Part model, mm, in its own coordinate system. Face numbers are marked on the shaded views. A direction names the side the tool comes from. Coordinates: 2 decimals unless noted, no trailing zeros. Order: outer loops, then holes, each group sorted by start corner. A loop starts at its lowest first (then second) coordinate and runs counter-clockwise, first axis right, second up.
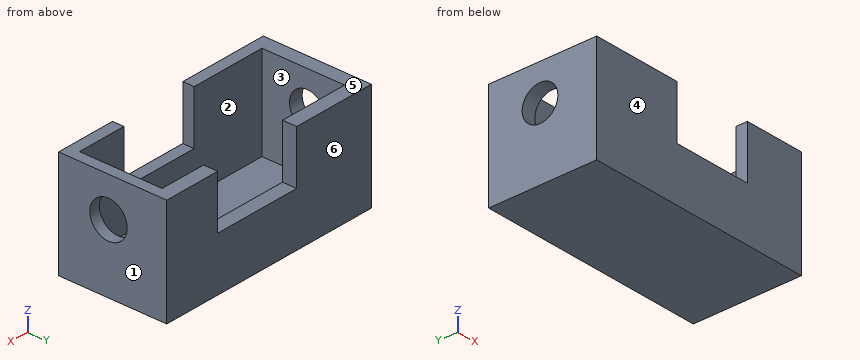
```python
from build123d import *

# Parameters (mm, degrees)
F0_W     = 218.6504378915
F0_H     = 102.5099009275
F1_DEPTH = 101.6
F2_W     = 194.8913782835
F2_H     = 78.3294849098
F3_DEPTH = 88.9
F4_W     = 84.4324864447
F4_H     = 13.4305804968
F4_W_2   = 74.9933160841
F4_H_2   = 10.749835521
F5_DEPTH = 50.8
F6_R     = 16.9313597919
F7_DEPTH = 25.4
F8_R     = 17.7291047607
F9_DEPTH = 25.4


with BuildPart() as f1:
    # F0 (on Top) → F1 (new body)
    with BuildSketch(Plane.XY):
        with Locations((-0.1867227256, -2.5207363069)):
            Rectangle(F0_W, F0_H)
    extrude(amount=F1_DEPTH)

    # F2 (on face) → F3 (cut)
    with BuildSketch(Plane.XY.offset(101.6)):
        with Locations((1.4596879482, -3.8611087948)):
            Rectangle(F2_W, F2_H)
    extrude(amount=-F3_DEPTH, mode=Mode.SUBTRACT)

    # F4 (on face) → F5 (cut)
    with BuildSketch(Plane.XY.offset(101.6)):
        with Locations((12.4733056873, 42.0189239085)):
            Rectangle(F4_W, F4_H)
        with Locations((13.9715243131, -48.4007690102)):
            Rectangle(F4_W_2, F4_H_2)
    extrude(amount=-F5_DEPTH, mode=Mode.SUBTRACT)

    # F6 (on face) → F7 (cut)
    with BuildSketch(Plane(origin=(-109.5119416714, 0, 0), x_dir=(0, -1, 0), z_dir=(-1, 0, 0))):
        with Locations((0, 67.3742890358)):
            Circle(F6_R)
    extrude(amount=-F7_DEPTH, mode=Mode.SUBTRACT)

    # F8 (on face) → F9 (cut)
    with BuildSketch(Plane.YZ.offset(109.1384962201)):
        with Locations((-6.4566782676, 64.2816573381)):
            Circle(F8_R)
    extrude(amount=-F9_DEPTH, mode=Mode.SUBTRACT)


solid = f1.part
```
(1) Pull direction Y, two halves, no side cores. Call the marked faces 3, 4, 5 and 6: +Y half, -Y half, draft (parallel to the pull), parting line (faces both ways), or undercut.
(2) Tool access for the marked faces 1 and 2: list every direction of +Z, -Z, +X, -X, +Y, -Y with a clear straight run to the whole face (end or side of a thin tool).
(3) Slice it at B-B, the plane y = -37.5. Give the cut face in (x, z), then the cut area to 3 significant figures.
(4) Slice it at D-D, the plane z = 30. Give the cut face in (x, y).
(5) Drop flat-ended pins along their axis: pin 1 (1.5 mm diameter, centred on y = 1, z = 77.5, fed in from -X); pin 2 (6.5 mm diameter, centred on x = -4, y = 45, fed in from +Z). Give the stop position or say it passes through.
(6) Slice it at C-C, the plane x = 40. Give the cut face in (y, z).
(7) Probe line 1 (Z direction, x = -104, y = 0); line 2 (Y direction, x = -69.5, z = 48); line 3 (X direction, y = 5, z = 20). List the from-to ranges inside material, lowest first.
(8) Slice it at A-A, the plane z = 73.5. Give the cut face in (x, y).
Here are the results:
1. face 3: undercut
1. face 4: -Y half
1. face 5: draft
1. face 6: +Y half
2. face 1: +Z, -Z, +X, +Y, -Y
2. face 2: +Z
3. outline: (-109.51, 0) - (109.14, 0) - (109.14, 101.6) - (98.91, 101.6) - (98.91, 12.7) - (-95.99, 12.7) - (-95.99, 101.6) - (-109.51, 101.6) - close
3. area: 4,890 mm2
4. outline: (-109.51, -53.78) - (109.14, -53.78) - (109.14, 48.73) - (-109.51, 48.73) - close; hole (-95.99, -43.03) - (98.91, -43.03) - (98.91, 35.3) - (-95.99, 35.3) - close
5. pin 1: passes through
5. pin 2: stops at z = 50.8
6. outline: (-53.78, 0) - (48.73, 0) - (48.73, 50.8) - (35.3, 50.8) - (35.3, 12.7) - (-43.03, 12.7) - (-43.03, 50.8) - (-53.78, 50.8) - close
7. line 1: z = 0 to 50.44, 84.31 to 101.6
7. line 2: y = -53.78 to -43.03, 35.3 to 48.73
7. line 3: x = -109.51 to -95.99, 98.91 to 109.14
8. outline: (-109.51, -53.78) - (-23.53, -53.78) - (-23.53, -43.03) - (-95.99, -43.03) - (-95.99, -15.78) - (-109.51, -15.78) - close; (-109.51, 15.78) - (-95.99, 15.78) - (-95.99, 35.3) - (-29.74, 35.3) - (-29.74, 48.73) - (-109.51, 48.73) - close; (51.47, -53.78) - (109.14, -53.78) - (109.14, -21.6) - (98.91, -21.6) - (98.91, -43.03) - (51.47, -43.03) - close; (54.69, 35.3) - (98.91, 35.3) - (98.91, 8.69) - (109.14, 8.69) - (109.14, 48.73) - (54.69, 48.73) - close
